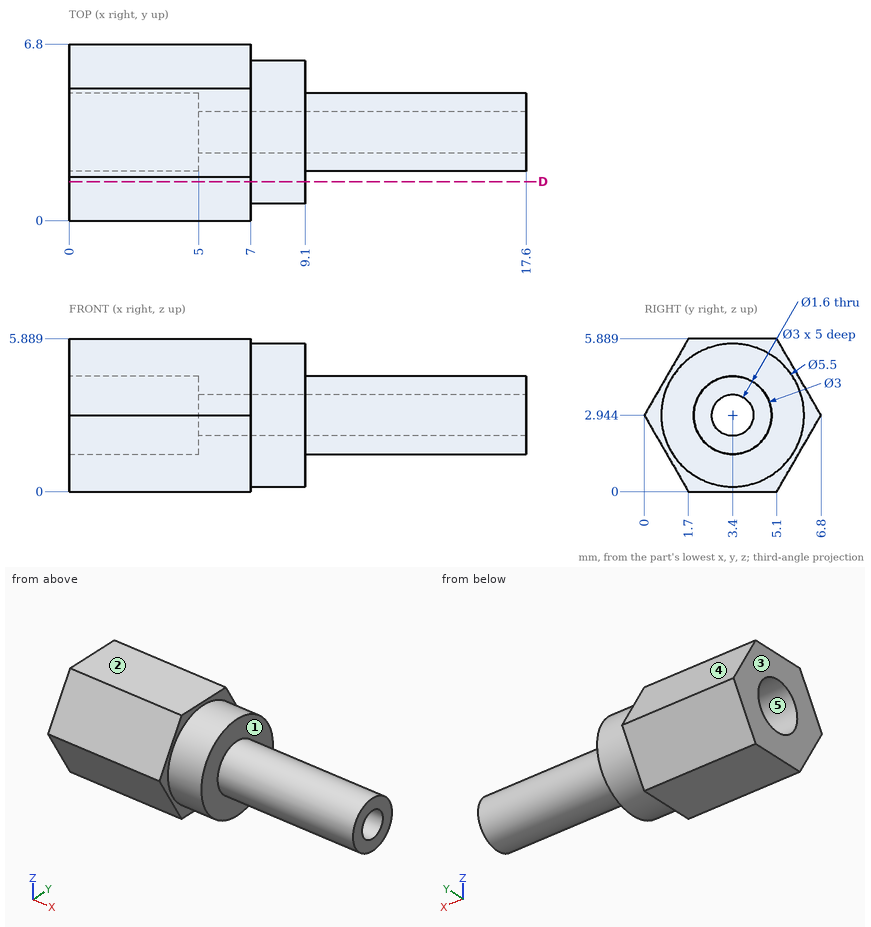
Study the drawing (mm; zero at the part's minimum x, y, z) and answer. A direction names the side the tool comes from. Round coordinates to 2 decimals unless told otherwise and drop trailing zeros. Loops run counter-clockwise (first coordinate to the right, second up) from the corner with the lowest first, then second, coordinate; pieces in that order, holes last. Notation, with made-up numbers: (12.5, 37.25) -> (27.5, 37.25) arc R28 ccw to (27.5, 71.25) -> close; hole circle Ø3 at (-5, -35). An arc over 180 degrees is marked (long way). Use one line per item in the form item = value.
1. Find the intervals of material crossed by probe 1 along X at (y, z) = (5.75, 1.75); probe 2 along X at (y, z) = (4.25, 3.85); probe 3 along Y at (x, z) = (10, 3.15) (1 decimal), in increasing order. Write a range as [from, to].
Answer key:
probe_1 = [0, 9.1]
probe_2 = [5, 17.6]
probe_3 = [1.9, 2.6], [4.2, 4.9]
2. Flat-ended cylindrical pins translate along their axes: pin 1 Ø1 at (x, y) = (13, 4) entering from +Z; pin 2 Ø1.5 at (x, y) = (7.5, 0.5) entering from +Z (1 decimal); pin 3 Ø3 at (y, z) = (3.5, 3.5) entering from +X; pin 4 Ø1 at (y, z) = (3.4, 2.94) entering from -X. Find the tip coordinate at first contact, or state that the pin passes through.
Answer key:
pin_1 = 4.44
pin_2 = 4.8
pin_3 = 17.6
pin_4 = through
3. The part is cut by section D-D on y = 1.5. Determine the outline of the cut face in (x, z).
Answer key:
outline = (0, 0.35) -> (7, 0.35) -> (7, 0.96) -> (9.1, 0.96) -> (9.1, 4.93) -> (7, 4.93) -> (7, 5.54) -> (0, 5.54) -> close
4. For a pull along Y with two mould halves and no side action, classify the marked faces 3, 4 and 5 as released by +Y, released by -Y, zero draft, split by the parting line, or undercut.
Answer key:
face_3 = zero draft
face_4 = released by +Y
face_5 = undercut
5. A tool of negligible diameter and unlimited length cuts with its end or side. For the marked faces 1 and 2, from which of +Z, -Z, +X, -X, +Y, -Y can it reach the whole face along a straight path? Write none if from no direction.
Answer key:
face_1 = +X
face_2 = +Z, +X, -X, +Y, -Y
